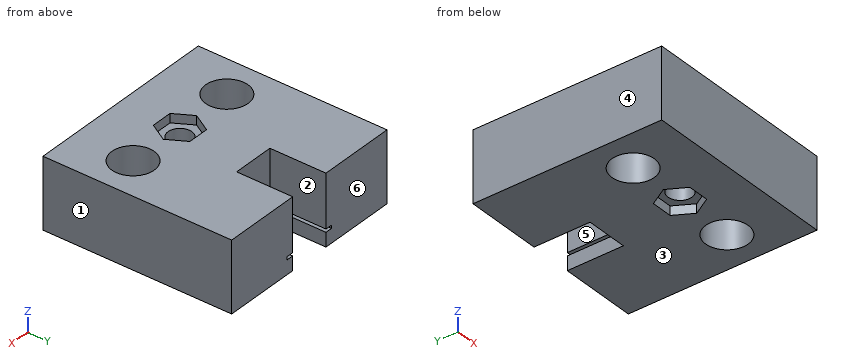
```python
from build123d import *

# Parameters (mm, degrees)
BOSS_EXTRUDE1_DEPTH     = 25
CUT_EXTRUDE1_DEPTH      = 3.2
CUT_EXTRUDE2_DEPTH      = 3.2
CUT_EXTRUDE3_DEPTH      = 62.39542258
CUT_EXTRUDE3_DEPTH_BACK = 62.39542258
SKETCH4_R               = 4.25
CUT_EXTRUDE4_DEPTH      = 63.603178144
CUT_EXTRUDE4_DEPTH_BACK = 63.603178144
SKETCH5_R               = 7.55
CUT_EXTRUDE5_DEPTH      = 20


with BuildPart() as part:
    # Sketch1 → Boss-Extrude1 (new body)
    with BuildSketch(Plane.XY):
        Polygon((-3.843317972, 42.253456221), (31.156682028, 42.253456221), (31.156682028, -25.046543779), (-4.705317324, -25.046543779), (-38.843317972, -25.046543779), (-38.843317972, 42.253456221), align=None)
    extrude(amount=BOSS_EXTRUDE1_DEPTH)

    # Sketch2 → Cut-Extrude1 (cut)
    with BuildSketch(Plane.XY.offset(25)):
        Polygon((3.679556035, -3.896543779), (-0.081880969, 2.618456221), (-7.604754976, 2.618456221), (-11.36619198, -3.896543779), (-7.604754976, -10.411543779), (-0.081880969, -10.411543779), align=None)
    extrude(amount=-CUT_EXTRUDE1_DEPTH, mode=Mode.SUBTRACT)

    # Sketch3 → Cut-Extrude2 (cut)
    with BuildSketch(Plane(origin=(0, 0, 0), x_dir=(-1, 0, 0), z_dir=(0, 0, -1))):
        Polygon((11.36619198, -3.896543779), (7.604754976, 2.618456221), (0.081880969, 2.618456221), (-3.679556035, -3.896543779), (0.081880969, -10.411543779), (7.604754976, -10.411543779), align=None)
    extrude(amount=-CUT_EXTRUDE2_DEPTH, mode=Mode.SUBTRACT)

    # Sketch4 → Cut-Extrude3 (cut, two sides: drawn at the far end of the back side and taken through both)
    with BuildSketch(Plane.XY.offset(21.8).offset(-CUT_EXTRUDE3_DEPTH_BACK)):
        with Locations((-3.843317972, -3.896543779)):
            Circle(SKETCH4_R)
    extrude(amount=CUT_EXTRUDE3_DEPTH + CUT_EXTRUDE3_DEPTH_BACK, mode=Mode.SUBTRACT)

    # Sketch5 → Cut-Extrude4 (cut, two sides: drawn at the far end of the back side and taken through both)
    with BuildSketch(Plane.XY.offset(25).offset(-CUT_EXTRUDE4_DEPTH_BACK)):
        with Locations((17.306682028, -3.896543779)):
            Circle(SKETCH5_R)
        with Locations(Location((-24.993317972, -3.896543779, 0), (0, 0, 180))):
            Circle(SKETCH5_R)
    extrude(amount=CUT_EXTRUDE4_DEPTH + CUT_EXTRUDE4_DEPTH_BACK, mode=Mode.SUBTRACT)

    # Sketch6 → Cut-Extrude5 (cut)
    with BuildSketch(Plane(origin=(0, 42.253456221, 0), x_dir=(1, 0, 0), z_dir=(0, 1, 0))):
        Polygon((-3.843317972, 0), (3.656682028, 0), (3.656682028, -5), (6.156682028, -5), (6.156682028, -6.1), (3.656682028, -6.1), (3.656682028, -25), (-11.343317972, -25), (-11.343317972, -6.1), (-13.843317972, -6.1), (-13.843317972, -5), (-11.343317972, -5), (-11.343317972, 0), align=None)
    extrude(amount=-CUT_EXTRUDE5_DEPTH, mode=Mode.SUBTRACT)


solid = part.part
```
Input: part model. Units: mm. Frame: model coordinates. Face numbers are marked on the shaded views. A direction names the side the tool comes from. Round coordinates to 2 decimals unless told otherwise and drop trailing zeros. Loops run counter-clockwise (first coordinate to the right, second up) from the corner with the lowest first, then second, coordinate; pieces in that order, holes last.
1) Pin query (flat end, axial travel): pin 1 (3 mm diameter, centred on x = -13, y = 31.5, fed in from -Z); pin 2 (2.5 mm diameter, centred on x = -3, z = 23, fed in from +Y); pin 3 (4 mm diameter, centred on x = -1, y = -7, fed in from +Z). Return the tip coordinate at first contact, or that it passes through.
Ans:
pin 1: stops at z = 0
pin 2: stops at y = 22.25
pin 3: stops at z = 21.8
2) Section query C-C on y = -0.5. Return the cut outline in (x, z), plus the area to 3 significant figures.
Ans:
outline: (-38.84, 0) - (-31.74, 0) - (-31.74, 25) - (-38.84, 25) - close; (-18.25, 0) - (-9.41, 0) - (-9.41, 3.2) - (-6.4, 3.2) - (-6.4, 21.8) - (-9.41, 21.8) - (-9.41, 25) - (-18.25, 25) - close; (-1.29, 3.2) - (1.72, 3.2) - (1.72, 0) - (10.56, 0) - (10.56, 25) - (1.72, 25) - (1.72, 21.8) - (-1.29, 21.8) - close; (24.05, 0) - (31.16, 0) - (31.16, 25) - (24.05, 25) - close
area: 909 mm2
3) Section query A-A on y = 30. Return the cut outline in (x, z).
Ans:
outline: (-38.84, 0) - (-11.34, 0) - (-11.34, 5) - (-13.84, 5) - (-13.84, 6.1) - (-11.34, 6.1) - (-11.34, 25) - (-38.84, 25) - close; (3.66, 0) - (31.16, 0) - (31.16, 25) - (3.66, 25) - (3.66, 6.1) - (6.16, 6.1) - (6.16, 5) - (3.66, 5) - close
4) Material intervals for line 1 (X direction, y = 36, z = 11.5); line 2 (X direction, y = -8, z = 22.25); line 3 (X direction, y = -2.5, z = 21.75), sorted ascending.
Ans:
line 1: x = -38.84 to -11.34, 3.66 to 31.16
line 2: x = -38.84 to -31.33, -18.66 to -9, 1.31 to 10.97, 23.64 to 31.16
line 3: x = -38.84 to -32.41, -17.57 to -7.86, 0.17 to 9.89, 24.73 to 31.16
5) Pull-direction query (X, two-part tool) for the marked faces 1, 2, 3 and 4; classes: released by +X, released by -X, zero draft, split by the parting line, or undercut.
Ans:
face 1: released by +X
face 2: undercut
face 3: zero draft
face 4: released by -X
6) Section query D-D on x = -1. Return the cut outline in (y, z).
Ans:
outline: (-25.05, 0) - (-10.41, 0) - (-10.41, 3.2) - (-7.06, 3.2) - (-7.06, 21.8) - (-10.41, 21.8) - (-10.41, 25) - (-25.05, 25) - close; (-0.74, 3.2) - (2.62, 3.2) - (2.62, 0) - (22.25, 0) - (22.25, 25) - (2.62, 25) - (2.62, 21.8) - (-0.74, 21.8) - close
7) Set-up query: the marked faces 5 and 6. Return all of +Z, -Z, +X, -X, +Y, -Y with unobstructed straight access to the full face (end or side cutting, diameter ignored); none if empty.
Ans:
face 5: +Z, -Z, +Y
face 6: +Z, -Z, +X, -X, +Y
8) Section query B-B on z = 12. Return the cut outline in (x, y).
Ans:
outline: (-38.84, -25.05) - (31.16, -25.05) - (31.16, 42.25) - (3.66, 42.25) - (3.66, 22.25) - (-11.34, 22.25) - (-11.34, 42.25) - (-38.84, 42.25) - close; hole circle Ø15.1 at (-24.99, -3.9); hole circle Ø8.5 at (-3.84, -3.9); hole circle Ø15.1 at (17.31, -3.9)
